from build123d import *

# Parameters (mm, degrees)
PAD003_DEPTH    = 2.5
POCKET004_DEPTH = 22.5
POCKET005_DEPTH = 10.013736


with BuildPart() as part:
    # Sketch010 → Pad003 (new body)
    with BuildSketch(Plane.XZ):
        with BuildLine():
            Line((-4.84295, 0), (4.84295, 0))
            Line((4.84295, 0), (4.84295, 22.5))
            Line((4.84295, 22.5), (5, 84))
            ThreePointArc((5, 84), (0, 89), (-5, 84))
            Line((-4.84295, 22.5), (-5, 84))
            Line((-4.84295, 22.5), (-4.84295, 0))
        make_face()
    extrude(amount=PAD003_DEPTH)

    # Sketch011 (on Face1 of Pad003) → Pocket004 (cut)
    with BuildSketch(Plane(origin=(0, 0, 0), x_dir=(1, 0, 0), z_dir=(0, 0, -1))):
        Polygon((-3.84295, 2.5), (-3.84295, 1), (-8.84295, 1), (-8.84295, 6.001038), align=None)
        Polygon((8.84295, 6.001038), (3.84295, 2.5), (3.84295, 1), (8.84295, 1), align=None)
    extrude(amount=-POCKET004_DEPTH, mode=Mode.SUBTRACT)

    # Sketch012 (on Face12 of Pocket004) → Pocket005 (cut, through all)
    with BuildSketch(Plane(origin=(-4.785462, 0, -0.01222), x_dir=(0.002554, 0, -0.999997), z_dir=(-0.999997, 0, -0.002554))):
        Polygon((-89.412494, 0.4), (-22.512294, 2.5), (-89.412494, 14.23), align=None)
    extrude(amount=-POCKET005_DEPTH, mode=Mode.SUBTRACT)


with BuildPart() as part_1:
    # Body001 placement: moved
    add(part.part.moved(Location((0, 25, 0))))


solid = part_1.part
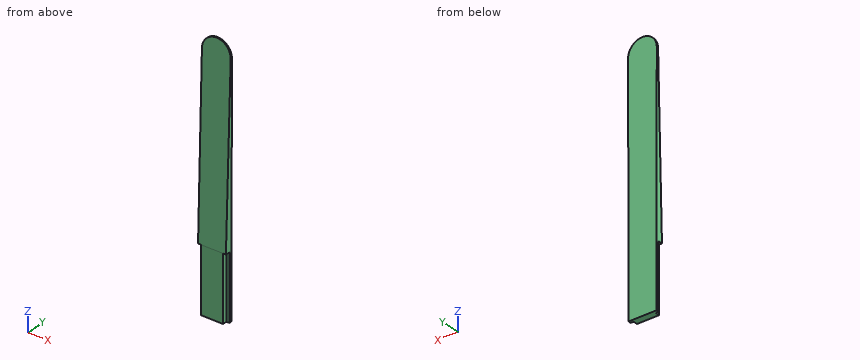
Verification items for the finished model (mm, model axes). Give positions to 0.01 mm unless a question says otherwise; leave off trailing zeros. Write each loop counter-clockwise with the first axis right and the second up, starting at its lowest first coordinate (ties: lowest second). Pieces come first, ordered by that corner, then holes. Notation, with made-up numbers: (38, 12.25) -> (83, 12.25) arc R28 cw to (83, 39.25) -> close; hole circle Ø3 at (-11.75, -15). An arc over 180 degrees is marked (long way). Use CSV: the item, a comma, the result in double quotes.
(1) Sectioned sample at B-B (z = 81.5). Record the cut outline in (x, y), plus the area to 3 significant figures.
Derived:
outline,"(-4.99, 24.35) -> (4.99, 24.35) -> (4.99, 25) -> (-4.99, 25) -> close"
area,"6.48 mm^2"
(2) Sectioned sample at A-A (x = 0). Record the cut outline in (y, z), plus the area to 3 significant figures.
Derived:
outline,"(22.5, 0) -> (25, 0) -> (25, 89) -> (24.59, 89) -> (22.5, 22.51) -> close"
area,"153 mm^2"
(3) Go/stop test with flat-tipped pins: pin 1 (1.2 mm diameter, centred on y = 23.5, z = 9, fed in from -X); pin 2 (1.2 mm diameter, centred on y = 23, z = 14, fed in from +X); pin 3 (0.5 mm diameter, centred on x = -4.5, z = 12, fed in from -Y). Record where each tip stops, or that it passes through.
Derived:
pin 1,"stops at x = -4.84"
pin 2,"stops at x = 3.84"
pin 3,"stops at y = 24"
(4) Material ranges on L1, parallel to X at y = 22.8, z = 12; L2, parallel to Y at x = 0.75, z = 70.5; L3, parallel to Y at x = -1.25, z = 84, recorded low to high.
Derived:
L1,"x = -3.84 to 3.84"
L2,"y = 24.01 to 25"
L3,"y = 24.43 to 25"
(5) Sectioned sample at C-C (z = 57.5). Record the cut outline in (x, y), plus the area to 3 significant figures.
Derived:
outline,"(-4.93, 23.6) -> (4.93, 23.6) -> (4.93, 25) -> (-4.93, 25) -> close"
area,"13.8 mm^2"
